```python
from build123d import *

# Parameters (mm, degrees)
F0_W     = 812.8
F0_H     = 762
F2_DEPTH = 127
F1_W     = 685.8
F1_H     = 635
F3_DEPTH = 215.9
F4_R     = 25.4


with BuildPart() as f2:
    # F0 (on Top) → F2 (new body)
    with BuildSketch(Plane.XY):
        Rectangle(F0_W, F0_H)
    extrude(amount=F2_DEPTH)

    # F1 (on face) → F3 (cut)
    with BuildSketch(Plane.XY):
        Rectangle(F1_W, F1_H)
    extrude(amount=F3_DEPTH, mode=Mode.SUBTRACT)

    # F4
    f4_edges = [f2.edges().sort_by_distance(p)[0] for p in [
        (406.4, 0, 127),
        (0, 381, 127),
        (-406.4, 0, 127),
        (0, -381, 127),
        (-406.4, 0, 0),
        (-406.4, -381, 63.5),
        (-406.4, 381, 63.5),
        (406.4, -381, 63.5),
        (406.4, 381, 63.5),
        (406.4, 0, 0),
        (0, 381, 0),
        (0, -381, 0),
    ]]
    fillet(f4_edges, radius=F4_R)


solid = f2.part
```
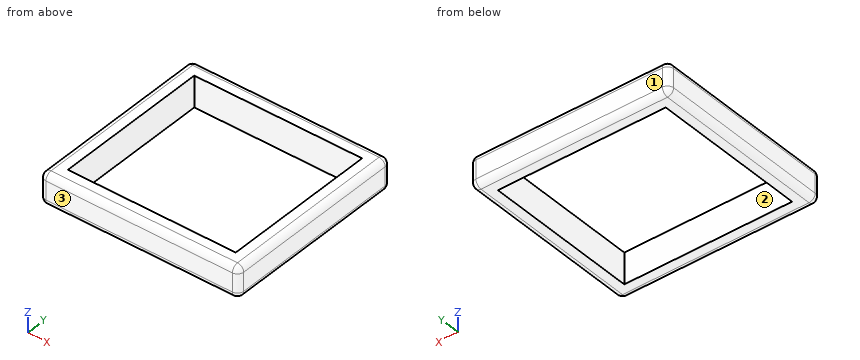
Verification items for the finished model (mm, model axes). Face numbers are marked on the shaded views. Coordinates: 2 decimals unless noted, no trailing zeros. Loops run counter-clockwise (first coordinate to the right, second up) from the corner with the lowest first, then second, coordinate; pieces in that order, holes last. Notation, with made-up numbers: (5, 41.5) - (63, 41.5) arc R29 cw to (63, 69.5) - close; hole circle Ø8 at (85, 17). An arc over 180 degrees is marked (long way). Put each result on its own line as item: value.
Item 1: Draft check along Y on the marked faces 1, 2 and 3. Enter one of: pulls with the +Y half, pulls with the -Y half, needs draft (parallel to the pull), parting line crosses it, or undercut.
Conclusion:
face 1: pulls with the +Y half
face 2: undercut
face 3: pulls with the -Y half
Item 2: Section check A-A (y = 69). Enter the section's corners in (x, z), then the cut area to 3 significant figures.
Conclusion:
outline: (-406.4, 25.4) arc R25.4 ccw to (-381, 0) - (-342.9, 0) - (-342.9, 127) - (-381, 127) arc R25.4 ccw to (-406.4, 101.6) - close; (342.9, 0) - (381, 0) arc R25.4 ccw to (406.4, 25.4) - (406.4, 101.6) arc R25.4 ccw to (381, 127) - (342.9, 127) - close
area: 15,600 mm2
Item 3: Section check C-C (z = 84). Enter the section's corners in (x, y), then the cut area to 3 significant figures.
Conclusion:
outline: (-406.4, -355.6) arc R25.4 ccw to (-381, -381) - (381, -381) arc R25.4 ccw to (406.4, -355.6) - (406.4, 355.6) arc R25.4 ccw to (381, 381) - (-381, 381) arc R25.4 ccw to (-406.4, 355.6) - close; hole (-342.9, -317.5) - (342.9, -317.5) - (342.9, 317.5) - (-342.9, 317.5) - close
area: 183,000 mm2
Item 4: Gauge pin test, flat end, axial feed: pin 1 Ø8 at (x, z) = (73.5, 17.5) entering from +Y. Record the tip position at first contact, or that the pin passes through.
Conclusion:
pin 1: stops at y = 380.7
Item 5: Section check B-B (x = -151). Enter the section's corners in (y, z).
Conclusion:
outline: (-381, 25.4) arc R25.4 ccw to (-355.6, 0) - (-317.5, 0) - (-317.5, 127) - (-355.6, 127) arc R25.4 ccw to (-381, 101.6) - close; (317.5, 0) - (355.6, 0) arc R25.4 ccw to (381, 25.4) - (381, 101.6) arc R25.4 ccw to (355.6, 127) - (317.5, 127) - close
Item 6: Scan lines: line 1 along Y through (x, z) = (19, 26); line 2 along X through (y, z) = (11, 92); line 3 along X through (y, z) = (-35, 21.5). Record each from-to range of solid material in increasing order.
Conclusion:
line 1: y = -381 to -317.5, 317.5 to 381
line 2: x = -406.4 to -342.9, 342.9 to 406.4
line 3: x = -406.1 to -342.9, 342.9 to 406.1
